Input: dimensioned drawing with shaded views. Units: mm. Origin: part minimum x, y, z. Round coordinates to 2 decimals unless told otherwise and drop trailing zeros. Loops run counter-clockwise (first coordinate to the right, second up) from the corner with the lowest first, then second, coordinate; pieces in that order, holes last. Notation, with made-up numbers: M 7.25,43.25 L 51.25,43.25 A28 cw 51.25,66.25 Z; hole C -14.5,-2 d1. An arc over 180 degrees is marked long. Answer as a JSON object with one key per item and string values.
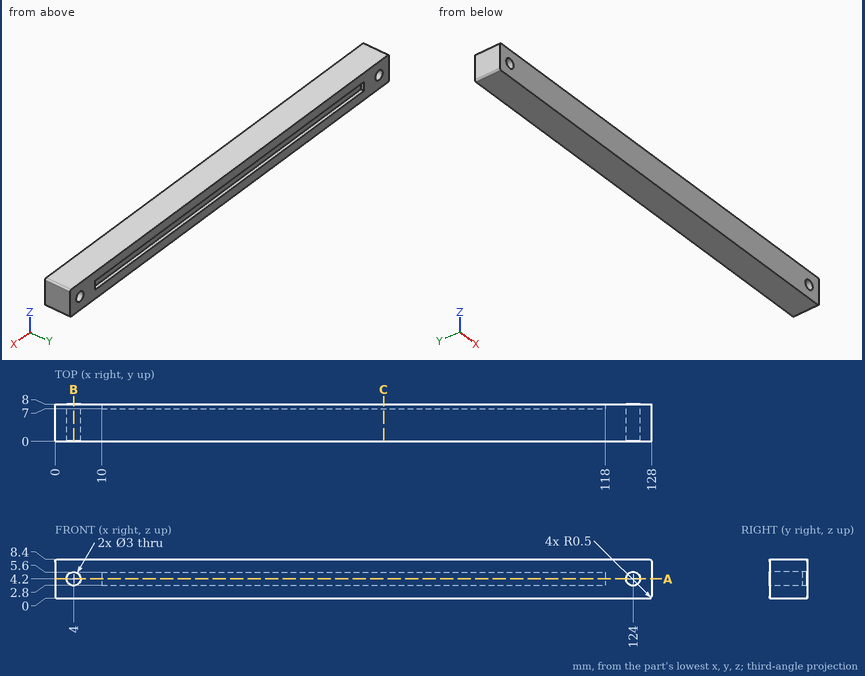
Item 1: Section C-C on x = 70.5. Return the cut outline in (y, z), then the cut area to 3 significant figures.
Answer sheet:
{"outline": "M 0,0 L 8,0 L 8,2.8 L 7,2.8 L 7,5.6 L 8,5.6 L 8,8.4 L 0,8.4 Z", "area": "64.4 mm²"}
Item 2: Section A-A on z = 4.2. Return the cut outline in (x, y), then the cut area to 3 significant figures.
Answer sheet:
{"outline": "M 0,0 L 2.5,0 L 2.5,8 L 0,8 Z; M 5.5,0 L 122.5,0 L 122.5,8 L 118,8 L 118,7 L 10,7 L 10,8 L 5.5,8 Z; M 125.5,0 L 128,0 L 128,8 L 125.5,8 Z", "area": "868 mm²"}
Item 3: Line query: probe 1 along X at (y, z) = (2.5, 4.2); probe 2 along Z at (x, y) = (124, 2); probe 3 along X at (y, z) = (3.25, 3.5). Output: solid intervals per line, ascending. Write a range as from..to.
Answer sheet:
{"probe 1": "x = 0..2.5, 5.5..122.5, 125.5..128", "probe 2": "z = 0..2.7, 5.7..8.4", "probe 3": "x = 0..2.67, 5.33..122.67, 125.33..128"}
Item 4: Section B-B on x = 4. Return the cut outline in (y, z), then the cut area to 3 significant figures.
Answer sheet:
{"outline": "M 0,0 L 8,0 L 8,2.7 L 0,2.7 Z; M 0,5.7 L 8,5.7 L 8,8.4 L 0,8.4 Z", "area": "43.2 mm²"}
Item 5: Contact query for flat-ended pins moving along their axis: pin 1 Ø0.5 at (x, y) = (88, 7.5) entering from -Z; pin 2 Ø2 at (x, z) = (37.5, 4.5) entering from +Y. Output: stop coordinate, or through.
Answer sheet:
{"pin 1": "stops at z = 0", "pin 2": "stops at y = 7"}
